Autodesk Inventor part; units mm, degrees
ref_plane "YZ Plane" through (0, 0, 0) normal (1, 0, 0) x (0, 1, 0)
ref_plane "XZ Plane" through (0, 0, 0) normal (0, 1, 0) x (-1, 0, 0)
ref_plane "XY Plane" through (0, 0, 0) normal (0, 0, 1) x (1, 0, 0)
sketch "Sketch1" plane through (0, 0, 0) normal (0, 0, 1) x (1, 0, 0)
  line L0 (-15, 0) -> (-6.35, 0)
  line L1 (-6.35, 0) -> (-6.35, 15)
  line L2 (-6.35, 15) -> (-7.5, 15)
  line L3 (-7.5, 15) -> (-7.5, 3)
  line L4 (-7.5, 3) -> (-15, 3)
  line L5 (-15, 3) -> (-15, 0)
  line L6 (0, -3) -> (0, 18)
  point P0 (0, 0)
  dimension "d0" = 3
  dimension "d2" = 15
  dimension "d3" = 6.35
  dimension "d4" = 15
  dimension "d17" = 7.5
  dimension "d18" = 1.15
revolve "Revolution1" add sketch "Sketch1" angle 360 about axis through (0, -10, 0) along (0, 1, 0)
sketch "Sketch2" plane through (0, 3, 0) normal (0, 1, 0) x (1, 0, 0)
  point P0 (0, 0)
  point P1 (0.0472, 12)
  dimension "d6" = 12
hole "Hole1" at (0.0472, 3, -12) direction (0, -1, 0) diameter 2.459 end through all
sketch "Sketch3" plane through (0, 15, 0) normal (0, 1, 0) x (1, 0, 0)
  line L0 (-15, 0.5) -> (15, 0.5)
  line L1 (15, 0.5) -> (15, -15)
  line L2 (15, -15) -> (-15, -15)
  line L3 (-15, -15) -> (-15, 0.5)
  circle A0 centre (0, 0) radius 15
  line L4 (-15, 0) -> (-7.5, 0)
  line L5 (-7.5, 0) -> (-7.5, 15)
  line L6 (-7.5, 15) -> (-15, 15)
  line L7 (-15, 15) -> (-15, 0)
  circle A1 centre (0, 0) radius 7.5
  line L8 (15, 0) -> (7.5, 0)
  line L9 (7.5, 0) -> (7.5, 15)
  line L10 (7.5, 15) -> (15, 15)
  line L11 (15, 15) -> (15, 0)
  point P0 (14.9917, 0.5)
  point P1 (-14.9917, 0.5)
  point P2 (7.5, 0.5)
  point P3 (-7.5, 0.5)
  point P4 (-7.5, 12.9904)
  dimension "d14" = 0.5
extrude "Extrusion1" cut sketch "Sketch3" against normal through all contours A0 L5 L0 | L0 L5 L4 A0 | A0 L2 L3 | L4 A1 L8 A0 | L0 A1 L5 | A0 L1 L2 | A1 L0 | L9 L10 L11 L0 A0 | A0 L0 L9 | L8 L9 L0 A0 | A1 L0 L9 picked at (-1.4202, -1.7241)
properties part number "BaffleClamp" material "Brass, Soft Yellow"
For this review, take the finished solid that the model builds, in its own axes (mm). A direction names the side the tool comes from. Give positions to 0.01 mm unless a question says otherwise; leave off trailing zeros. Write each loop counter-clockwise with the first axis right and the second up, starting at its lowest first coordinate (ties: lowest second). Pieces come first, ordered by that corner, then holes. Notation, with made-up numbers: M 34.5,51.5 L 78.5,51.5 A17 cw 78.5,82.5 Z; hole C 58.5,48 d10. An arc over 180 degrees is marked long. Answer as a JSON object with one key per item and string values. Group by question number.
Item 1: Consider section B-B on x = -0.25. Write out the cut boundary in (y, z), plus the area to 3 significant figures.
Item 2: Tool access review of faces 1 (the cylindrical face through (0, 1, -15)), 2 (the cylindrical face through (-0.16, 8.92, -7.5)): name each direction out of +Z, -Z, +X, -X, +Y, -Y from which nothing blocks a thin tool from reaching the whole face with its end or side.
Item 3: For pin 1 Ø3 at (y, z) = (5.5, -5.5) entering from +X; pin 2 Ø6 at (x, y) = (2, 12) entering from +Z; pin 3 Ø6 at (x, z) = (-3, -12) entering from +Y, all flat-tipped, find the tip position at first contact; note any pin that passes through.
Item 4: Draft analysis for pull direction X (two halves, no side actions). For faces 3 (the flat face through (7.5, 2, -7)), 4 (the flat face through (0, 15, -7)), 5 (the cylindrical face through (-0.322, 1.479, -10.827)), state which applies: +X half, -X half, draft (parallel to the pull), parting line (faces both ways), or undercut.
Item 5: Consider section A-A on z = -12. Write out the cut boundary in (x, y), plus the area to 3 significant figures.
Item 6: Consider section D-D on x = 4. Write out the cut boundary in (y, z).
Item 7: Consider section C-C on z = -8.75. Write out the cut boundary in (x, y).
Item 8: For probe 1 along X at (y, z) = (0.75, -12); probe 2 along Y at (x, z) = (5.25, -7.25); probe 3 along X at (y, z) = (10.25, -1.75), list the stretches that pass through material, from the lowest coordinate up. Write a range as [from, to].
Check result:
{
 "1": {"outline": "M 0,-15 L 3,-15 L 3,-13.19 L 0,-13.19 Z; M 0,-10.81 L 3,-10.81 L 3,-7.5 L 15,-7.5 L 15,-6.35 L 0,-6.35 Z", "area": "32.6 mm^2"},
 "2": {"face 1": "-Z, +Y, -Y", "face 2": "-Z, +Y"},
 "3": {"pin 1": "stops at x = 6.34", "pin 2": "stops at z = -3.91", "pin 3": "stops at y = 3"},
 "4": {"face 3": "+X half", "face 4": "draft", "face 5": "undercut"},
 "5": {"outline": "M -7.5,0 L -1.18,0 L -1.18,3 L -7.5,3 Z; M 1.28,0 L 7.5,0 L 7.5,3 L 1.28,3 Z", "area": "37.6 mm^2"},
 "6": {"outline": "M 0,-14.46 L 3,-14.46 L 3,-6.34 L 15,-6.34 L 15,-4.93 L 0,-4.93 Z"},
 "7": {"outline": "M -7.5,0 L 7.5,0 L 7.5,3 L -7.5,3 Z"},
 "8": {"probe 1": "x = [-7.5, -1.18], [1.28, 7.5]", "probe 2": "y = [0, 3]", "probe 3": "x = [-7.29, -6.1], [6.1, 7.29]"}
}
